Source: CAD feature listing. Evaluate the final solid. Frame: model axes, mm. A direction names the side the tool comes from. Give positions to 0.01 mm unless a question says otherwise; leave off trailing zeros. Order: outer loops, then holes, each group sorted by start corner. A loop starts at its lowest first (then second) coordinate and runs counter-clockwise, first axis right, second up.
from build123d import *

# Parameters (mm, degrees)
SKETCH1_R           = 17
SKETCH1_R_2         = 9.5
BOSS_EXTRUDE1_DEPTH = 10
SKETCH2_R           = 20
SKETCH2_R_2         = 9.5
BOSS_EXTRUDE2_DEPTH = 8
CHAMFER1_SIZE       = 2
FILLET1_R           = 2


with BuildPart() as part:
    # Sketch1 → Boss-Extrude1 (new body)
    with BuildSketch(Plane.XY):
        Circle(SKETCH1_R)
        Circle(SKETCH1_R_2, mode=Mode.SUBTRACT)
    extrude(amount=BOSS_EXTRUDE1_DEPTH)

    # Sketch2 → Boss-Extrude2 (add)
    with BuildSketch(Plane.XY.offset(10)):
        Circle(SKETCH2_R)
        Circle(SKETCH2_R_2, mode=Mode.SUBTRACT)
    extrude(amount=BOSS_EXTRUDE2_DEPTH)

    # Chamfer1
    chamfer1_edges = [part.edges().sort_by_distance(p)[0] for p in [
        (-9.5, 0, 0),
    ]]
    chamfer(chamfer1_edges, length=CHAMFER1_SIZE)

    # Fillet1
    fillet1_edges = [part.edges().sort_by_distance(p)[0] for p in [
        (-9.5, 0, 2),
    ]]
    fillet(fillet1_edges, radius=FILLET1_R)


solid = part.part
(1) Section A-A, the plane y = 16. Return loops of the section in (x, z), plus the area to 3 significant figures.
(2) Section C-C, the plane x = 15. Return loops of the section in (y, z), plus the area to 3 significant figures.
(3) Section B-B, the plane z = 13. Return loops of the section in (x, y), plus the area to 3 significant figures.
(4) Line query: line 1 along Y through (x, z) = (0, 7.5); line 2 along Y through (x, z) = (0, 14); line 3 along X through (y, z) = (-8.5, 10.25). Output: solid intervals per line, ascending.
(5) Pin query (flat end, axial travel): pin 1 Ø1 at (x, z) = (-13.5, 12) entering from +Y; pin 2 Ø1.5 at (x, z) = (13.5, 13) entering from -Y; pin 3 Ø6 at (y, z) = (16, 11) entering from +X. Return the tip coordinate at first contact, or that it passes through.
(6) Access query for faces 4 (the flat face through (4, -9, 18)), 5 (the cylindrical face through (9.139, 14.334, 4.93)). Directions: +Z, -Z, +X, -X, +Y, -Y. A direction counts if a zero-diameter tool reaches every point of the face in a straight line with its end or side. Return the directions, or none.
(7) Draft query along X for faces 1 (the cylindrical face through (4.38, -8.43, 10.31)), 2 (the flat face through (-9, -15, 10)), 3 (the cylindrical face through (-4.336, -19.524, 13.944)). Return one class per face: +X half, -X half, draft (parallel to the pull), parting line (faces both ways), or undercut.
(8) Section D-D, the plane z = 4.25. Return loops of the section in (x, y), plus the area to 3 significant figures.
Checks:
1. outline: (-12, 10) - (-5.74, 10) - (-5.74, 0) - (5.74, 0) - (5.74, 10) - (12, 10) - (12, 18) - (-12, 18) - close
1. area: 307 mm2
2. outline: (-13.23, 10) - (-8, 10) - (-8, 0) - (8, 0) - (8, 10) - (13.23, 10) - (13.23, 18) - (-13.23, 18) - close
2. area: 372 mm2
3. outline: circle Ø40 at (0, 0); hole circle Ø19 at (0, 0)
3. area: 973 mm2
4. line 1: y = -17 to -9.5, 9.5 to 17
4. line 2: y = -20 to -9.5, 9.5 to 20
4. line 3: x = -18.1 to -4.24, 4.24 to 18.1
5. pin 1: stops at y = 15.2
5. pin 2: stops at y = -15.41
5. pin 3: stops at x = 15.2
6. face 4: +Z, +X, -X, +Y, -Y
6. face 5: -Z
7. face 1: undercut
7. face 2: draft
7. face 3: parting line
8. outline: circle Ø34 at (0, 0); hole circle Ø19 at (0, 0)
8. area: 624 mm2
